Solid Edge part; units mm, degrees
sketch "Sketch1" plane through (0, 0, 0) normal (-1, 0, 0) x (0, -1, 0)
  line L0 (23.6, 20.423) -> (29.1, 20.423)
  line L1 (29.1, 20.423) -> (29.1, 22.423)
  line L2 (29.1, 22.423) -> (29.1, 36.173)
  line L3 (29.1, 36.173) -> (24.6, 36.173)
  line L4 (24.6, 36.173) -> (24.6, 34.173)
  line L5 (24.6, 34.173) -> (26.6, 34.173)
  line L6 (26.6, 34.173) -> (27.1, 22.423)
  line L7 (23.6, 22.423) -> (27.1, 22.423)
  line L8 (23.6, 20.423) -> (23.6, 22.423)
  dimension "D1" = 29.1
  dimension "D2" = 29.1
  dimension "D3" = 23.6
  dimension "D4" = 23.6
  dimension "D5" = 24.6
  dimension "D6" = 29.1
  dimension "D7" = 24.6
  dimension "D8" = 23.6
revolve "RevolvedProtrusion1" add sketch "Sketch1" angle 360 about axis through (0, 0, 57) along (0, 0, -1)
sketch "Sketch2" plane through (0, 0, 0) normal (-1, 0, 0) x (0, -1, 0)
  line L0 (-20.1, 36.173) -> (-20.1, 25.173)
  line L1 (-20.1, 25.173) -> (20.1, 25.173)
  line L2 (20.1, 25.173) -> (20.1, 36.173)
  line L3 (20.1, 36.173) -> (-20.1, 36.173)
  dimension "D1" = 20.1
extrude "Cutout1" cut sketch "Sketch2" along normal mid plane 75
sketch "Sketch3" plane through (0, 0, 0) normal (0, -1, 0) x (1, 0, 0)
  line L0 (-12.0428, 36.173) -> (-12.0428, 25.173)
  line L1 (-12.0428, 25.173) -> (12.0428, 25.173)
  line L2 (12.0428, 25.173) -> (12.0428, 36.173)
  line L3 (12.0428, 36.173) -> (-12.0428, 36.173)
  dimension "D1" = 12.0428
  dimension "D2" = 12.0428
extrude "Extrusionsausschnitt_2" cut sketch "Sketch3" along normal mid plane 75
fillet "Verrundung_0_5_mm" radius 0.5 12 edges at (19.5224, -20.1, 25.173) (-12.0428, -25.3188, 25.173) (12.0428, -25.3188, 25.173) (-19.5224, -20.1, 25.173) (-19.5224, 20.1, 25.173) (-12.0428, 25.3188, 25.173) (12.0428, 25.3188, 25.173) (19.5224, 20.1, 25.173) (14.8434, 22.0734, 34.173) (-14.8434, 22.0734, 34.173) (-14.8434, -22.0734, 34.173) (14.8434, -22.0734, 34.173)
fillet "Verrundung_0_75_mm" radius 0.75 4 edges at (-16.8486, -23.7262, 36.173) (16.8486, -23.7262, 36.173) (16.8486, 23.7262, 36.173) (-16.8486, 23.7262, 36.173)
Source: CAD feature listing. Evaluate the final solid. Frame: model axes, mm. A direction names the side the tool comes from. Give positions to 0.01 mm unless a question says otherwise; leave off trailing zeros. Order: outer loops, then holes, each group sorted by start corner. A loop starts at its lowest first (then second) coordinate and runs counter-clockwise, first axis right, second up. Notation, with made-up numbers: (52.25, -20.75) -> (61.25, -20.75) arc R9 cw to (61.25, -10.75) -> close; hole circle Ø4 at (-38, -17). An arc over 180 degrees is marked (long way). Use a Markdown table: item, result.
1) Contact query for flat-ended pins moving along their axis: P1, Ø1.5, axis at y = 25, z = 28.5, coming from the +X side; P2, Ø2.5, axis at x = -4.5, y = 27, coming from the +Z side; P3, Ø2, axis at x = -22, y = -12, coming from the +Z side. Output: stop coordinate, or through.
Answer list:
| item | result |
|---|---|
| P1 | x = 16.09 |
| P2 | z = 25.17 |
| P3 | z = 22.42 |
2) Section query A-A, the plane x = 0. Return the cut outline in (y, z).
Answer list:
| item | result |
|---|---|
| outline | (-29.1, 20.42) -> (-23.6, 20.42) -> (-23.6, 22.42) -> (-27.1, 22.42) -> (-26.98, 25.17) -> (-29.1, 25.17) -> close; (23.6, 20.42) -> (29.1, 20.42) -> (29.1, 25.17) -> (26.98, 25.17) -> (27.1, 22.42) -> (23.6, 22.42) -> close |
3) Section query B-B, the plane z = 31.25. Return the cut outline in (x, y), then the cut area to 3 significant figures.
Answer list:
| item | result |
|---|---|
| outline | (-21.04, -20.1) arc R29.1 ccw to (-12.04, -26.49) -> (-12.04, -23.86) arc R26.72 cw to (-17.61, -20.1) -> close; (-21.04, 20.1) -> (-17.61, 20.1) arc R26.72 cw to (-12.04, 23.86) -> (-12.04, 26.49) arc R29.1 ccw to start; (12.04, -26.49) arc R29.1 ccw to (21.04, -20.1) -> (17.61, -20.1) arc R26.72 cw to (12.04, -23.86) -> close; (12.04, 23.86) arc R26.72 cw to (17.61, 20.1) -> (21.04, 20.1) arc R29.1 ccw to (12.04, 26.49) -> close |
| area | 85.0 mm² |
4) Reachability of faces 4 (the conical face through (-17.6, 20.36, 26.78)), 5 (the cylindrical face through (-13.15, 20.79, 35.16)), 6 (the flat face through (-18, -20.1, 32)), 7 (the flat face through (12.043, -24, 32)) from +Z, -Z, +X, -X, +Y, -Y: full face, straight path, thin tool, end or side. Return the list, or none.
Answer list:
| item | result |
|---|---|
| face 4 | none |
| face 5 | +Z |
| face 6 | +Z, +X, -X |
| face 7 | +Z, +Y, -Y |
5) Ray query, line 1 along Y through (x, z) = (0, 21.7); line 2 along Z through (x, y) = (-22.5, 12.5). Return the intervals inside material, ascending. Write a range as [from, to].
Answer list:
| item | result |
|---|---|
| line 1 | [-29.1, -23.6], [23.6, 29.1] |
| line 2 | [20.42, 22.42] |
6) Mould query, pull axis X, two halves, no side actions, for faces 1 (the cylindrical face through (13.15, -20.79, 35.16)), 2 (the flat face through (-15, -22, 36.173)), 3 (the cylindrical face through (1.28, 29.07, 24.69)). Classes: +X half, -X half, draft (parallel to the pull), parting line (faces both ways), or undercut.
Answer list:
| item | result |
|---|---|
| face 1 | undercut |
| face 2 | draft |
| face 3 | parting line |
